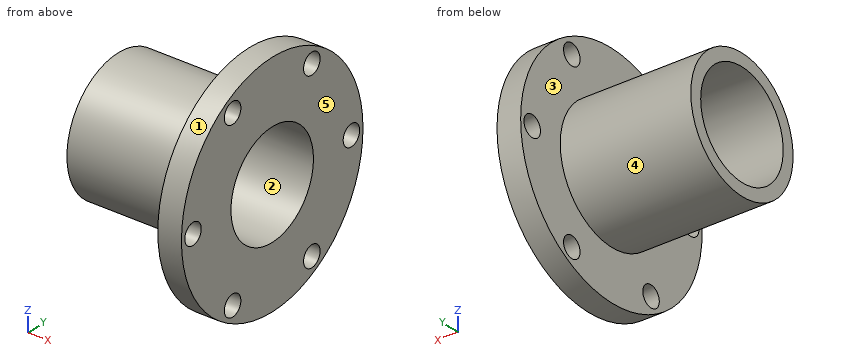
```python
from build123d import *

# Parameters (mm, degrees)
SKETCH2_R          = 10
CUT_EXTRUDE1_DEPTH = 30
CIRPATTERN1_COUNT  = 6


with BuildPart() as part:
    # Sketch1 → Revolve1 (revolve)
    with BuildSketch(Plane.XY):
        Polygon((-147.64573991, 50), (0, 50), (0, 110), (-22.64573991, 110), (-22.64573991, 62), (-147.64573991, 62), align=None)
    revolve(axis=Axis((-203.3632287, 0, 0), (1, 0, 0)))

    # Sketch2 → Cut-Extrude1 (cut)
    with BuildSketch(Plane(origin=(0, 0, 0), x_dir=(0, 0, -1), z_dir=(1, 0, 0))):
        with Locations((0, 96)):
            Circle(SKETCH2_R)
    cut_extrude1 = extrude(amount=-CUT_EXTRUDE1_DEPTH, mode=Mode.SUBTRACT)

    # CirPattern1: Cut-Extrude1 ×6 about axis
    cirpattern1_axis = Axis((0, 0, 0), (1, 0, 0))
    for i in range(1, CIRPATTERN1_COUNT):
        add(cut_extrude1.rotate(cirpattern1_axis, i * 360 / CIRPATTERN1_COUNT), mode=Mode.SUBTRACT)


solid = part.part
```
Here's how the part is built. I have some questions about the finished solid (model axes, mm). Face numbers are marked on the shaded views. A direction names the side the tool comes from. Coordinates: 2 decimals unless noted, no trailing zeros. Write each loop counter-clockwise with the first axis right and the second up, starting at its lowest first coordinate (ties: lowest second). Pieces come first, ordered by that corner, then holes. Notation, with made-up numbers: (-38.5, -2.5) -> (-31.5, -2.5) arc R14 ccw to (-31.5, 18.5) -> close; hole circle Ø11 at (34, 3). An arc over 180 degrees is marked (long way). Use a Markdown table: item, result. Add a question column.
(1) If we section it at D-D, the plane x = -18: Write out the boundary of the cut face in (y, z), and give its area (3 significant figures).
(2) If we section it at B-B, the plane x = -135: Write out the boundary of the cut face in (y, z), and give its area (3 significant figures).
(3) Please list where these lines run through material, in increasing order: line 1 (Y direction, x = -8, z = -1); line 2 (Z direction, x = -106.5, y = 0); line 3 (X direction, y = -94, z = 15).
(4) We'd pull the mould along Z, two halves only. Please class the marked faces 1, 2 and 3: +Z half, -Z half, draft (parallel to the pull), parting line (faces both ways), or undercut.
(5) I'm going to push flat-ended pins straight in: P1, Ø1.5, axis at x = -96, y = -46, coming from the -Z side; P2, Ø1, axis at x = -122.5, z = -41.5, coming from the -Y side; P3, Ø8, axis at x = -92.5, z = 46.5, coming from the +Y side. Where does each tip first touch, or does it pass through?
(6) If we section it at C-C, the plane z = -27: Write out the boundary of the cut face in (x, y), and give its area (3 significant figures).
(7) If we section it at A-A, the plane y = 0: Write out the boundary of the cut face in (x, z), and give its area (3 significant figures).
(8) For the marked faces 4 and 5, which set-ups out of +Z, -Z, +X, -X, +Y, -Y let a thin tool reach every point of the face, with its end or its side?
Outcome:
| question | item | result |
|---|---|---|
| 1 | outline | circle Ø220 at (0, 0); hole circle Ø20 at (-96, 0); hole circle Ø20 at (-48, -83.14); hole circle Ø20 at (-48, 83.14); hole circle Ø100 at (0, 0); hole circle Ø20 at (48, -83.14); hole circle Ø20 at (48, 83.14); hole circle Ø20 at (96, 0) |
| 1 | area | 28,300 mm^2 |
| 2 | outline | circle Ø124 at (0, 0); hole circle Ø100 at (0, 0) |
| 2 | area | 4,220 mm^2 |
| 3 | line 1 | y = -110 to -105.95, -86.05 to -49.99, 49.99 to 86.05, 105.95 to 110 |
| 3 | line 2 | z = -62 to -50, 50 to 62 |
| 3 | line 3 | x = -22.65 to 0 |
| 4 | face 1 | parting line |
| 4 | face 2 | undercut |
| 4 | face 3 | draft |
| 5 | P1 | stops at z = -42.38 |
| 5 | P2 | stops at y = -46.51 |
| 5 | P3 | stops at y = 45.14 |
| 6 | outline | (-147.65, -55.81) -> (-22.65, -55.81) -> (-22.65, -106.63) -> (0, -106.63) -> (0, -42.08) -> (-147.65, -42.08) -> close; (-147.65, 42.08) -> (0, 42.08) -> (0, 106.63) -> (-22.65, 106.63) -> (-22.65, 55.81) -> (-147.65, 55.81) -> close |
| 6 | area | 6,360 mm^2 |
| 7 | outline | (-147.65, -62) -> (-22.65, -62) -> (-22.65, -110) -> (0, -110) -> (0, -50) -> (-147.65, -50) -> close; (-147.65, 50) -> (0, 50) -> (0, 110) -> (-22.65, 110) -> (-22.65, 62) -> (-147.65, 62) -> close |
| 7 | area | 5,720 mm^2 |
| 8 | face 4 | -X |
| 8 | face 5 | +Z, -Z, +X, +Y, -Y |
